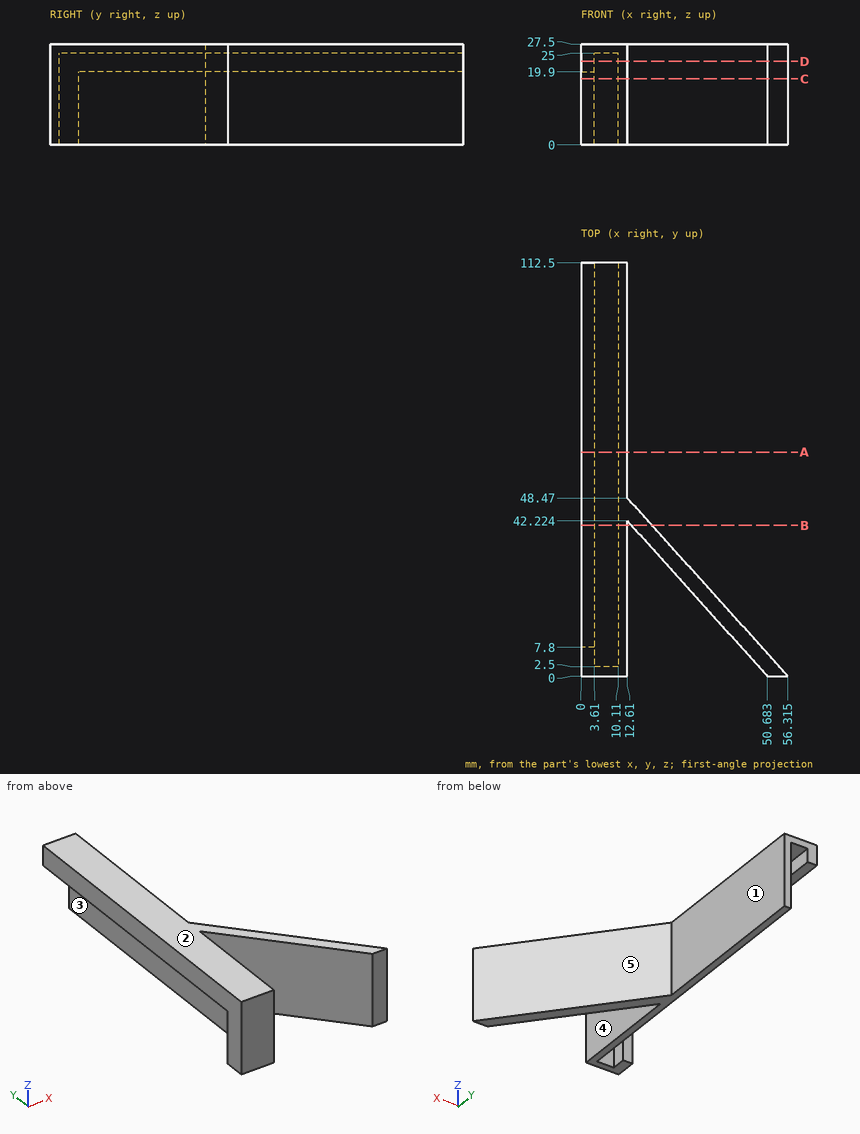
Answer from the drawing. Dimensions are ordinates in mm from the lowest x, y and z of the part. A direction names the side the tool comes from. Coordinates: 2 decimals unless noted, no trailing zeros. Write each loop counter-clockwise with the first axis right and the second up, starting at its lowest first coordinate (ties: lowest second). Pieces come first, ordered by that corner, then holes. Notation, with made-up numbers: M 74.25,-23.5 L 99.25,-23.5 A25 ccw 99.25,14.5 Z; hole C -4,20 d8. An arc over 180 degrees is marked long. Use a Markdown table: item, result.
Q1. Which of the six approach directions +Z, -Z, +X, -X, +Y, -Y give full straight-line access (tool end or side, diameter ignored) to the marked faces 4 and 5?
Answer block:
| item | result |
|---|---|
| face 4 | +Z, -Z, -Y |
| face 5 | +Z, -Z, +X, +Y |
Q2. The part is cut by section C-C, the plane z = 18. Write down the section's boundary in (x, y) (1 decimal), then the cut area to 3 significant figures.
Answer block:
| item | result |
|---|---|
| outline | M 0,0 L 12.6,0 L 12.6,42.2 L 50.7,0 L 56.3,0 L 12.6,48.5 L 12.6,112.5 L 10.1,112.5 L 10.1,2.5 L 3.6,2.5 L 3.6,7.8 L 0,7.8 Z |
| area | 581 mm2 |
Q3. Determine the mould class of the marked faces 1, 2 and 3 for opening direction X: released by +X, released by -X, zero draft, split by the parting line, or undercut.
Answer block:
| item | result |
|---|---|
| face 1 | released by +X |
| face 2 | zero draft |
| face 3 | undercut |
Q4. The part is cut by section B-B, the plane y = 41. Write down the section's boundary in (x, z) (1 decimal).
Answer block:
| item | result |
|---|---|
| outline | M 0,19.9 L 3.6,19.9 L 3.6,25 L 10.1,25 L 10.1,0 L 12.6,0 L 12.6,27.5 L 0,27.5 Z; M 13.7,0 L 19.3,0 L 19.3,27.5 L 13.7,27.5 Z |
Q5. Each of these flat-tipped pins is pushed along its axis until it touches: pin 1 Ø2 at (y, z) = (38, 6) entering from +X; pin 2 Ø4 at (y, z) = (44, 3.5) entering from -X; pin 3 Ø4 at (x, y) = (2, 59.5) entering from -Z. Where does it stop, or does it pass through?
Answer block:
| item | result |
|---|---|
| pin 1 | stops at x = 22.95 |
| pin 2 | stops at x = 10.11 |
| pin 3 | stops at z = 19.9 |
Q6. The part is cut by section A-A, the plane y = 61. Write down the section's boundary in (x, z).
Answer block:
| item | result |
|---|---|
| outline | M 0,19.9 L 3.61,19.9 L 3.61,25 L 10.11,25 L 10.11,0 L 12.61,0 L 12.61,27.5 L 0,27.5 Z |
Q7. The part is cut by section D-D, the plane z = 22.75. Write down the section's boundary in (x, y) (1 decimal).
Answer block:
| item | result |
|---|---|
| outline | M 0,0 L 12.6,0 L 12.6,42.2 L 50.7,0 L 56.3,0 L 12.6,48.5 L 12.6,112.5 L 10.1,112.5 L 10.1,2.5 L 3.6,2.5 L 3.6,112.5 L 0,112.5 Z |
Q8. Straight lines are drawn through the part: L1, parallel to X at y = 6.5, z = 24.25 (1 decimal); L2, parallel to Y at x = 7, z = 4.5; L3, parallel to X at y = 88, z = 12. For each, find the intervals that lie inside material, in ascending order. Write a range as [from, to].
Answer block:
| item | result |
|---|---|
| L1 | x = [0, 3.6], [10.1, 12.6], [44.8, 50.5] |
| L2 | y = [0, 2.5] |
| L3 | x = [10.11, 12.61] |
